Print and shaded views of the part. All mm, measured from the part's lowest x, y and z. A direction names the side the tool comes from. Give positions to 0.01 mm unless a question says otherwise; leave off trailing zeros. Loops run counter-clockwise (first coordinate to the right, second up) from the corner with the lowest first, then second, coordinate; pieces in that order, holes last. Notation, with made-up numbers: M 7.25,-11.75 L 53.25,-11.75 A24 ccw 53.25,2.25 Z; hole C 5.25,-31.5 d9. An arc over 180 degrees is marked long. Answer in a Markdown table with one row per item.
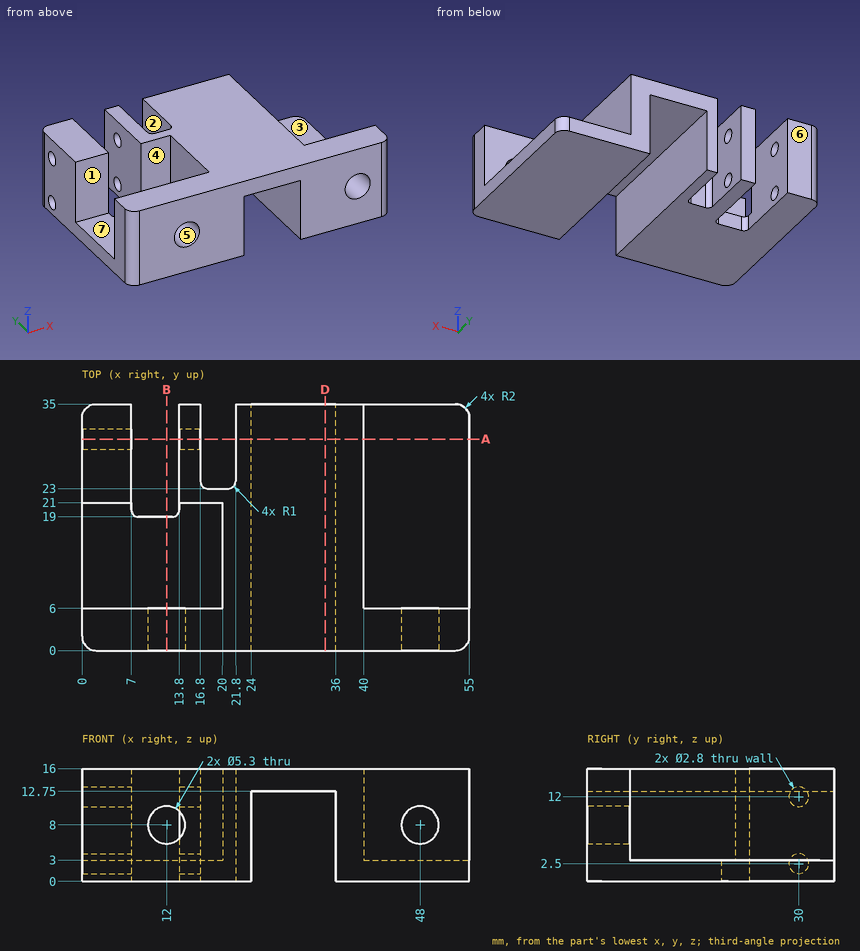
(1) Mould opens along Y. For the marked faces 4, 5, 6 and 7 say: pulls with the +Y half, pulls with the -Y half, needs draft (parallel to the pull), parting line crosses it, or undercut.
Established:
| item | result |
|---|---|
| face 4 | undercut |
| face 5 | needs draft |
| face 6 | pulls with the +Y half |
| face 7 | undercut |
(2) Which spindle directions (+Z, -Z, +X, -X, +Y, -Y) get a long thin tool onto all of the face, cutting with end or side? Do the marked faces 1, 2 and 3. Say none if no direction does.
Established:
| item | result |
|---|---|
| face 1 | +Z, -X |
| face 2 | +Z, -Z, +Y |
| face 3 | +Z, +X, +Y |
(3) Saw through at D-D, the plane x = 34.5. Give the cut face in (y, z).
Established:
| item | result |
|---|---|
| outline | M 0,12.75 L 35,12.75 L 35,16 L 0,16 Z |
(4) Flat gauge pins, fed straight in: P1, Ø4, axis at y = 13.5, z = 9.5, coming from the -X side; P2, Ø2.5, axis at y = 30, z = 12, coming from the +X side; P3, Ø8, axis at x = 29, y = 31, coming from the -Z side. Where does each tip first touch, or does it go through?
Established:
| item | result |
|---|---|
| P1 | stops at x = 20 |
| P2 | stops at x = 40 |
| P3 | stops at z = 12.75 |
(5) Saw through at B-B, the plane x = 12. Give the cut face in (y, z).
Established:
| item | result |
|---|---|
| outline | M 0,0 L 19,0 L 19,3 L 6,3 L 6,5.35 L 0,5.35 Z; M 0,10.65 L 6,10.65 L 6,16 L 0,16 Z |
(6) Saw through at A-A, the plane y = 30. Count the separate pieces of the cut face and the enclosed holes in it, and give its area (3 significant figures).
Established:
| item | result |
|---|---|
| separate pieces | 7 |
| enclosed holes | 0 |
| area | 287 mm2 |
(7) Wall check: L1, parallel to X at y = 22, z = 5.5; L2, parallel to X at y = 24.5, z = 9.5; L3, parallel to Z at x = 2.5, y = 30. Give the ranges that are in metal, low to high.
Established:
| item | result |
|---|---|
| L1 | x = 0 to 7, 13.8 to 24, 36 to 40 |
| L2 | x = 0 to 7, 13.8 to 16.8, 21.8 to 24, 36 to 40 |
| L3 | z = 0 to 1.1, 3.9 to 10.6, 13.4 to 16 |
